Check sheet for the modelled part. Datum: model origin and axes. Units: mm. A direction names the side the tool comes from. Round coordinates to 2 decimals unless told otherwise and drop trailing zeros. Write each loop counter-clockwise with the first axis right and the second up, starting at its lowest first coordinate (ties: lowest second). Pieces come first, ordered by that corner, then holes. Notation, with made-up numbers: M 88.25,-4.75 L 128.25,-4.75 A13 ccw 128.25,0.25 Z; hole C 2.25,-27 d2. An arc over 180 degrees is marked long. Put each result on its own line as item: value.
```python
from build123d import *

# Parameters (mm, degrees)
SKETCH_1_W          = 30
SKETCH_1_H          = 10
EXTRUDE_1_DEPTH     = 5
SKETCH_2_W          = 6.2
SKETCH_2_H          = 6
CUT_EXTRUDE_1_DEPTH = 2
SKETCH_3_R          = 1.5
CUT_EXTRUDE_4_DEPTH = 2
SKETCH_5_W          = 30
SKETCH_5_H          = 10
SKETCH_5_W_2        = 28
SKETCH_5_H_2        = 7
CUT_EXTRUDE_5_DEPTH = 4


with BuildPart() as part:
    # 草图1 → 凸台-拉伸1 (new body)
    with BuildSketch(Plane.XY):
        with Locations((-25.027311994, -7.227757648)):
            Rectangle(SKETCH_1_W, SKETCH_1_H)
    extrude(amount=EXTRUDE_1_DEPTH)

    # 草图2 → 切除-拉伸1 (cut)
    with BuildSketch(Plane(origin=(0, 0, 0), x_dir=(-1, 0, 0), z_dir=(0, 0, -1))):
        with Locations((21.488967254, -7.159562762)):
            Rectangle(SKETCH_2_W, SKETCH_2_H)
        with Locations((14.688967254, -7.159562762)):
            Rectangle(SKETCH_2_W, SKETCH_2_H)
        with Locations((28.288967254, -7.159562762)):
            Rectangle(SKETCH_2_W, SKETCH_2_H)
        with Locations((35.088967254, -7.159562762)):
            Rectangle(SKETCH_2_W, SKETCH_2_H)
    extrude(amount=-CUT_EXTRUDE_1_DEPTH, mode=Mode.SUBTRACT)

    # 草图3 → 切除-拉伸4 (cut)
    with BuildSketch(Plane(origin=(0, 0, 2), x_dir=(-1, 0, 0), z_dir=(0, 0, -1))):
        with Locations((14.688967254, -7.159562762)):
            Circle(SKETCH_3_R)
        with Locations((21.488967254, -7.159562762)):
            Circle(SKETCH_3_R)
        with Locations((28.288967254, -7.159562762)):
            Circle(SKETCH_3_R)
        with Locations((35.088967254, -7.159562762)):
            Circle(SKETCH_3_R)
    extrude(amount=-CUT_EXTRUDE_4_DEPTH, mode=Mode.SUBTRACT)

    # 草图5 → 切除-拉伸5 (cut)
    with BuildSketch(Plane.XY.offset(5)):
        with Locations((-25.027311994, -7.227757648)):
            Rectangle(SKETCH_5_W, SKETCH_5_H)
        with Locations((-24.3244943, -7.159562762)):
            Rectangle(SKETCH_5_W_2, SKETCH_5_H_2, mode=Mode.SUBTRACT)
    extrude(amount=-CUT_EXTRUDE_5_DEPTH, mode=Mode.SUBTRACT)


solid = part.part
```
1. Scan lines: probe 1 along X at (y, z) = (-6, 0.4); probe 2 along X at (y, z) = (-6.75, 3.75); probe 3 along Y at (x, z) = (-33.75, 1.5). Record each from-to range of solid material in increasing order.
Computed values:
probe 1: x = -40.03 to -38.19, -31.99 to -31.39, -25.19 to -24.59, -18.39 to -17.79, -11.59 to -10.03
probe 2: x = -38.32 to -36.53, -33.65 to -29.73, -26.85 to -22.93, -20.05 to -16.13, -13.25 to -10.32
probe 3: y = -10.66 to -10.16, -4.16 to -3.66
2. Access from +Z, -Z, +X, -X, +Y, -Y to the whole of each face (thin tool, end or side, straight path). Record for faces 1 (the flat face through (-20, -6, 2)), 2 (the flat face through (-29, -4, 0)), 3 (the flat face through (-38.324, -7, 3)).
Computed values:
face 1: -Z
face 2: -Z, +X, -X, +Y, -Y
face 3: +Z, -X, +Y, -Y
3. Cross-section at D-D (z = 4.4). Enter the section's corners in (x, y), then the cut area to 3 significant figures.
Computed values:
outline: M -38.32,-10.66 L -10.32,-10.66 L -10.32,-3.66 L -38.32,-3.66 Z
area: 196 mm2
4. Cross-section at A-A (z = 1.7). Enter the section's corners in (x, y).
Computed values:
outline: M -38.32,-10.66 L -10.32,-10.66 L -10.32,-3.66 L -38.32,-3.66 Z; hole M -38.19,-10.16 L -31.99,-10.16 L -31.99,-4.16 L -38.19,-4.16 Z; hole M -31.39,-10.16 L -25.19,-10.16 L -25.19,-4.16 L -31.39,-4.16 Z; hole M -24.59,-10.16 L -18.39,-10.16 L -18.39,-4.16 L -24.59,-4.16 Z; hole M -17.79,-10.16 L -11.59,-10.16 L -11.59,-4.16 L -17.79,-4.16 Z
5. Depth check by flat-ended pin: pin 1 Ø2 at (x, y) = (-35.5, -8) entering from -Z; pin 2 Ø1.5 at (y, z) = (-8, 4) entering from -X; pin 3 Ø0.9 at (x, y) = (-15, -6.5) entering from -Z. Enter the tip coordinate at first touch or a pass-through.
Computed values:
pin 1: stops at z = 2
pin 2: stops at x = -38.32
pin 3: stops at z = 4
6. Release check for a two-part mould opening along X. For faces 4 (the flat face through (-28, -4.16, 1)), 5 (the flat face through (-25, -7, 5)), 6 (the flat face through (-40.027, -7.3, 0.5)) record: +X half, -X half, draft (parallel to the pull), parting line (faces both ways), or undercut.
Computed values:
face 4: undercut
face 5: draft
face 6: -X half
7. Cross-section at B-B (y = -9.5). Enter the section's corners in (x, z).
Computed values:
outline: M -40.03,0 L -38.19,0 L -38.19,2 L -31.99,2 L -31.99,0 L -31.39,0 L -31.39,2 L -25.19,2 L -25.19,0 L -24.59,0 L -24.59,2 L -18.39,2 L -18.39,0 L -17.79,0 L -17.79,2 L -11.59,2 L -11.59,0 L -10.03,0 L -10.03,1 L -10.32,1 L -10.32,5 L -38.32,5 L -38.32,1 L -40.03,1 Z
8. Cross-section at C-C (z = 0.5). Enter the section's corners in (x, y).
Computed values:
outline: M -40.03,-12.23 L -10.03,-12.23 L -10.03,-2.23 L -40.03,-2.23 Z; hole M -38.19,-10.16 L -31.99,-10.16 L -31.99,-4.16 L -38.19,-4.16 Z; hole M -31.39,-10.16 L -25.19,-10.16 L -25.19,-4.16 L -31.39,-4.16 Z; hole M -24.59,-10.16 L -18.39,-10.16 L -18.39,-4.16 L -24.59,-4.16 Z; hole M -17.79,-10.16 L -11.59,-10.16 L -11.59,-4.16 L -17.79,-4.16 Z
